```python
from build123d import *

# Parameters (mm, degrees)
SKETCH1_R                = 2.75
BOSS_EXTRUDE1_DEPTH      = 2
SKETCH2_W                = 3
SKETCH2_H                = 100
BOSS_EXTRUDE2_DEPTH      = 2
SKETCH3_W                = 60
SKETCH3_H                = 3
BOSS_EXTRUDE3_DEPTH      = 2
CHAMFER1_SIZE            = 2
CHAMFER1_OF_MIRROR1_SIZE = 2


with BuildPart() as part:
    # Sketch1 → Boss-Extrude1 (new body)
    with BuildSketch(Plane(origin=(0, 0, 0), x_dir=(1, 0, 0), z_dir=(0, 1, 0))):
        Polygon((-17.5, 42.995), (-17.5, -42.995), (-36.7, -42.995), (-36.7, -109.005), (36.7, -109.005), (36.7, -42.995), (17.5, -42.995), (17.5, 42.995), (36.7, 42.995), (36.7, 109.005), (-36.7, 109.005), (-36.7, 42.995), align=None)
        with Locations(Location((-31.7, 102.855, 0), (0, 0, 270))):
            Circle(SKETCH1_R, mode=Mode.SUBTRACT)
        with Locations(Location((-31.7, 49.145, 0), (0, 0, 270))):
            Circle(SKETCH1_R, mode=Mode.SUBTRACT)
        with Locations(Location((31.7, 49.145, 0), (0, 0, 270))):
            Circle(SKETCH1_R, mode=Mode.SUBTRACT)
        with Locations(Location((31.7, 102.855, 0), (0, 0, 270))):
            Circle(SKETCH1_R, mode=Mode.SUBTRACT)
        with Locations(Location((31.7, -102.855, 0), (0, 0, 270))):
            Circle(SKETCH1_R, mode=Mode.SUBTRACT)
        with Locations(Location((31.7, -49.145, 0), (0, 0, 270))):
            Circle(SKETCH1_R, mode=Mode.SUBTRACT)
        with Locations(Location((-31.7, -49.145, 0), (0, 0, 270))):
            Circle(SKETCH1_R, mode=Mode.SUBTRACT)
        with Locations(Location((-31.7, -102.855, 0), (0, 0, 270))):
            Circle(SKETCH1_R, mode=Mode.SUBTRACT)
    extrude(amount=BOSS_EXTRUDE1_DEPTH)

    # Sketch2 → Boss-Extrude2 (add)
    with BuildSketch(Plane(origin=(0, 2, 0), x_dir=(1, 0, 0), z_dir=(0, 1, 0))):
        with Locations((12, -50)):
            Rectangle(SKETCH2_W, SKETCH2_H)
        with Locations((0, -50)):
            Rectangle(SKETCH2_W, SKETCH2_H)
        with Locations((-12, -50)):
            Rectangle(SKETCH2_W, SKETCH2_H)
    boss_extrude2 = extrude(amount=BOSS_EXTRUDE2_DEPTH)

    # Sketch3 → Boss-Extrude3 (add)
    with BuildSketch(Plane(origin=(0, 2, 0), x_dir=(1, 0, 0), z_dir=(0, 1, 0))):
        with Locations((0, -91)):
            Rectangle(SKETCH3_W, SKETCH3_H)
        with Locations((0, -61)):
            Rectangle(SKETCH3_W, SKETCH3_H)
        with Locations((0, -76)):
            Rectangle(SKETCH3_W, SKETCH3_H)
    boss_extrude3 = extrude(amount=BOSS_EXTRUDE3_DEPTH)

    # Chamfer1
    chamfer1_edges = [part.edges().sort_by_distance(p)[0] for p in [
        (30, 4, 61),
        (30, 4, 76),
        (30, 4, 91),
        (12, 4, 100),
        (0, 4, 100),
        (-12, 4, 100),
        (-30, 4, 91),
        (-30, 4, 76),
        (-30, 4, 61),
    ]]
    chamfer(chamfer1_edges, length=CHAMFER1_SIZE - 0.0001)  # a hair under: the kernel refuses the full size

    # Mirror1: Boss-Extrude2, Boss-Extrude3 across plane
    add(boss_extrude2.mirror(Plane.XY))
    add(boss_extrude3.mirror(Plane.XY))

    # Chamfer1 of Mirror1
    chamfer1_of_mirror1_edges = [part.edges().sort_by_distance(p)[0] for p in [
        (30, 4, -61),
        (30, 4, -76),
        (30, 4, -91),
        (12, 4, -100),
        (0, 4, -100),
        (-12, 4, -100),
        (-30, 4, -91),
        (-30, 4, -76),
        (-30, 4, -61),
    ]]
    chamfer(chamfer1_of_mirror1_edges, length=CHAMFER1_OF_MIRROR1_SIZE - 0.0001)  # a hair under: the kernel refuses the full size


solid = part.part
```
Check sheet for the modelled part. Datum: model origin and axes. Units: mm. A direction names the side the tool comes from. Give positions to 0.01 mm unless a question says otherwise; leave off trailing zeros. Write each loop counter-clockwise with the first axis right and the second up, starting at its lowest first coordinate (ties: lowest second). Pieces come first, ordered by that corner, then holes.
Item 1: Scan lines: L1, parallel to X at y = 2.15, z = 78; L2, parallel to Z at x = -15.5, y = 3.35; L3, parallel to Z at x = 28, y = 1.2 (3 decimals). Record each from-to range of solid material in increasing order.
Item 2: Cross-section at D-D (z = -49). Enter the section's corners in (x, y).
Item 3: Cross-section at B-B (z = -16). Enter the section's corners in (x, y).
Item 4: Gauge pin test, flat ends, axial feed: pin 1 (1.6 mm diameter, centred on y = 3.5, z = -85, fed in from -X); pin 2 (1.5 mm diameter, centred on y = 2.5, z = 26.5, fed in from +X); pin 3 (1.6 mm diameter, centred on y = 3, z = -97.5, fed in from +X). Record the tip position at first contact, or that the pin passes through.
Item 5: Cross-section at C-C (y = 0.6). Count the separate pieces of the cut face and the enclosed holes in it, and give its area (3 significant figures).
Item 6: Access from +Z, -Z, +X, -X, +Y, -Y to the whole of each face (thin tool, end or side, straight path). Record for faces 3 (the face through (32.526, 0.986, 105.478)), 4 (the face through (-17, 2, -2)).
Item 7: Draft check along X on faces 1 (the face through (-6, 2, -69)), 2 (the face through (0, 4, 0)). Enter one of: released by +X, released by -X, zero draft, split by the parting line, or undercut.
Report:
1. L1: x = -13.5 to -10.5, -1.5 to 1.5, 10.5 to 13.5
1. L2: z = -92.5 to -89.5, -77.5 to -74.5, -62.5 to -59.5, 59.5 to 62.5, 74.5 to 77.5, 89.5 to 92.5
1. L3: z = -109.005 to -42.995, 42.995 to 109.005
2. outline: (-36.7, 0) - (-34.45, 0) - (-34.45, 2) - (-36.7, 2) - close; (-28.95, 0) - (28.95, 0) - (28.95, 2) - (13.5, 2) - (13.5, 4) - (10.5, 4) - (10.5, 2) - (1.5, 2) - (1.5, 4) - (-1.5, 4) - (-1.5, 2) - (-10.5, 2) - (-10.5, 4) - (-13.5, 4) - (-13.5, 2) - (-28.95, 2) - close; (34.45, 0) - (36.7, 0) - (36.7, 2) - (34.45, 2) - close
3. outline: (-17.5, 0) - (17.5, 0) - (17.5, 2) - (13.5, 2) - (13.5, 4) - (10.5, 4) - (10.5, 2) - (1.5, 2) - (1.5, 4) - (-1.5, 4) - (-1.5, 2) - (-10.5, 2) - (-10.5, 4) - (-13.5, 4) - (-13.5, 2) - (-17.5, 2) - close
4. pin 1: stops at x = -13.5
4. pin 2: stops at x = 17.5
4. pin 3: stops at x = 13.5
5. separate pieces: 1
5. enclosed holes: 8
5. area: 12,500 mm2
6. face 3: +Y, -Y
6. face 4: +Y
7. face 1: undercut
7. face 2: zero draft
